from build123d import *

# Parameters (mm, degrees)
F0_R     = 32.5
F0_R_2   = 16.5
F1_DEPTH = 4
F2_R     = 1.99999


# Not quite as in the source:
# - a fillet or chamfer is up to 0.001 mm smaller than in the source, because OpenCascade refuses the exact size
# - a feature names something its author has since deleted; it is built from what else it names


with BuildPart() as f1:
    # F0 (on Front) → F1 (new body)
    with BuildSketch(Plane.XZ):
        Circle(F0_R)
        Circle(F0_R_2, mode=Mode.SUBTRACT)
    extrude(amount=F1_DEPTH)

    # F2 (radius 2 in the source; OpenCascade refuses exactly that, so slightly less here)
    f2_edges = [f1.edges().sort_by_distance(p)[0] for p in [
        (-32.5, -4, 0),
        (-32.5, 0, 0),
        (-16.5, 0, 0),
        (-16.5, -4, 0),
    ]]
    fillet(f2_edges, radius=F2_R)


solid = f1.part
Work out the finished part from the listing and answer in its coordinate system (mm). Give positions to 0.01 mm unless a question says otherwise; leave off trailing zeros. Write each loop counter-clockwise with the first axis right and the second up, starting at its lowest first coordinate (ties: lowest second). Pieces come first, ordered by that corner, then holes. Notation, with made-up numbers: M -27.5,8.5 L 18.5,8.5 A14 ccw 18.5,35.5 Z; hole C 69,33 d9. An arc over 180 degrees is marked long. Answer as CSV lines item,"result".
Q1. A cutting plane is placed at C-C on y = -3.1. Write down the section's boundary in (x, z).
A:
outline,"C 0,0 d64.34; hole C 0,0 d33.66"
Q2. Given P1, Ø8, axis at x = 4, z = 12.5, coming from the +Y side; P2, Ø1.5, axis at y = -2, z = -18.5, coming from the +X side, each flat-ended and moving along its own axis, determine where each tip first touches the part or whether it passes through.
A:
P1,"stops at y = -0.55"
P2,"stops at x = 27.22"
Q3. Find the intervals of material crossed by probe 1 along Z at (x, y) = (0, -2); probe 2 along Z at (x, y) = (15, -0.55); probe 3 along X at (y, z) = (-3.6, -4.5), in increasing order. Write a range as [from, to].
A:
probe 1,"z = [-32.5, -16.5], [16.5, 32.5]"
probe 2,"z = [-28.13, -8.26], [8.26, 28.13]"
probe 3,"x = [-31.38, -16.7], [16.7, 31.38]"
